Answer from the drawing. Dimensions are ordinates in mm from the lowest x, y and z of the part. A direction names the side the tool comes from. Give positions to 0.01 mm unless a question says otherwise; leave off trailing zeros. Loops run counter-clockwise (first coordinate to the right, second up) from the corner with the lowest first, then second, coordinate; pieces in that order, holes last. Notation, with made-up numbers: (-36, -31.75) - (-31, -31.75) arc R11 ccw to (-31, -19.75) - close; hole circle Ø3 at (46, 64). An arc over 180 degrees is marked (long way). Write each question's results on one line, items separated by ' | '. Start each with the question number.
Q1. The part is cut by section A-A, the plane z = 18.75. Write down the section's boundary in (x, y), plus the area to 3 significant figures.
Q2. The part is cut by section C-C, the plane x = 33. Write down the section's boundary in (y, z).
Q3. The part is cut by section D-D, the plane y = 48. Write down the section's boundary in (x, z), plus the area to 3 significant figures.
Q4. For the marked faces 1, 2, 3 and 4, determine the directions among +Z, -Z, +X, -X, +Y, -Y from which every point of the face is accessible in a straight line to the end or side of a thin tool.
Q5. Determine the mould class of the marked faces 5, 6 and 7 for opening direction Y: +Y half, -Y half, draft (parallel to the pull), parting line (faces both ways), or undercut.
Q6. The part is cut by section B-B, the plane y = 25. Write down the section's boundary in (x, z).
Q7. Given pin 1 (3 mm diameter, centred on y = 20, z = 21, fed in from +X); pin 2 (2 mm diameter, centred on x = 33, y = 62, fed in from +Z); pin 3 (1 mm diameter, centred on x = 9.5, y = 47.5, fed in from +Z); pin 4 (6 mm diameter, centred on x = 50.5, z = 15.5, fed in from +Y), each flat-ended and moving along its own axis, determine where each tip first touches the part or whether it passes through.
Q8. Find the intervals of material crossed by line 1 (Y direction, x = 33, z = 2); line 2 (Y direction, x = 32.5, z = 18); line 3 (Z direction, x = 46.5, y = 31), in increasing order. Write a range as from..to.
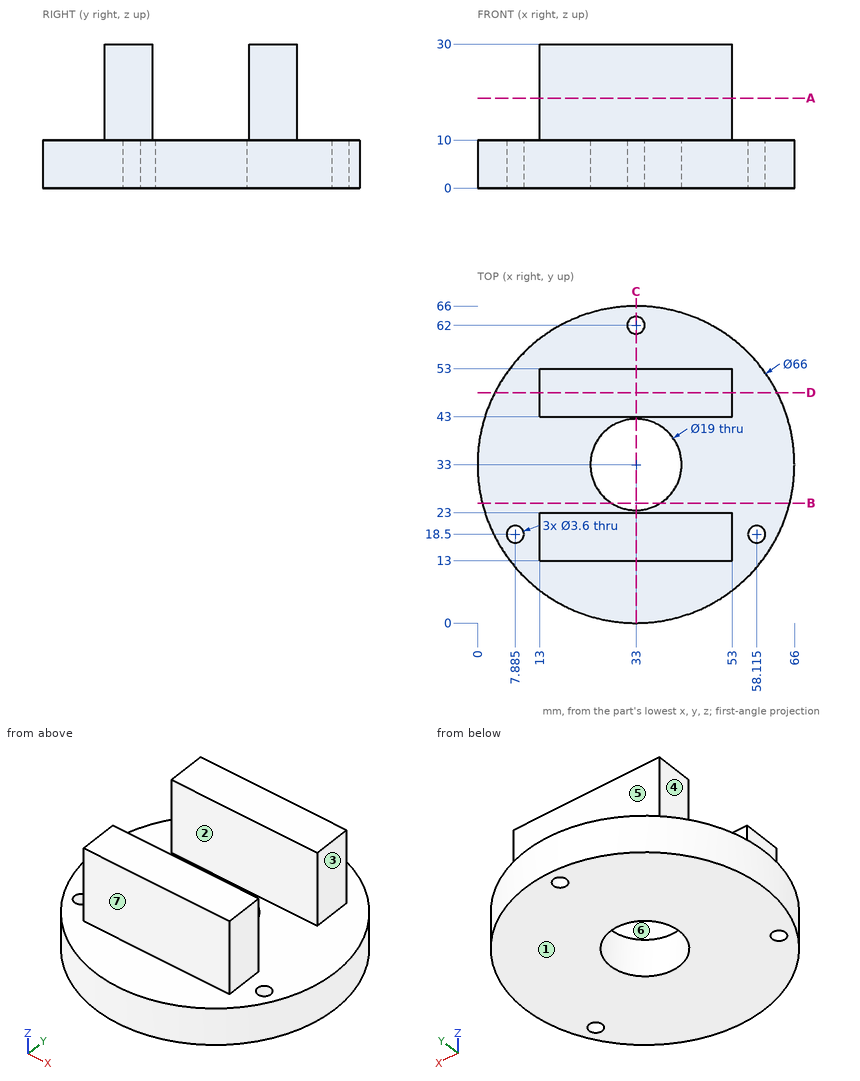
Check sheet entries:
1) outline: (13, 13) - (53, 13) - (53, 23) - (13, 23) - close; (13, 43) - (53, 43) - (53, 53) - (13, 53) - close | area: 800 mm^2
2) outline: (0, 0) - (23.5, 0) - (23.5, 10) - (23, 10) - (23, 30) - (13, 30) - (13, 10) - (0, 10) - close; (42.5, 0) - (60.2, 0) - (60.2, 10) - (53, 10) - (53, 30) - (43, 30) - (43, 10) - (42.5, 10) - close; (63.8, 0) - (66, 0) - (66, 10) - (63.8, 10) - close
3) outline: (3.61, 0) - (62.39, 0) - (62.39, 10) - (53, 10) - (53, 30) - (13, 30) - (13, 10) - (3.61, 10) - close | area: 1,390 mm^2
4) face 1: -Z, +X, -X, +Y, -Y | face 2: +Z, +X, -X | face 3: +Z, +X, +Y, -Y | face 4: +Z, -X, +Y, -Y
5) face 5: +Y half | face 6: undercut | face 7: -Y half
6) outline: (0.98, 0) - (27.88, 0) - (27.88, 10) - (0.98, 10) - close; (38.12, 0) - (65.02, 0) - (65.02, 10) - (38.12, 10) - close
7) pin 1: stops at x = 53 | pin 2: passes through | pin 3: stops at z = 10 | pin 4: stops at y = 53
8) line 1: y = 0..23.5, 42.5..60.2, 63.8..66 | line 2: y = 13..23, 43..53 | line 3: z = 0..10
